Here's how the part is built. I have some questions about the finished solid (model axes, mm). Coordinates: 2 decimals unless noted, no trailing zeros. Loops run counter-clockwise (first coordinate to the right, second up) from the corner with the lowest first, then second, coordinate; pieces in that order, holes last. Notation, with made-up numbers: M -24,49.25 L 1,49.25 A22 cw 1,83.25 Z; hole C -10,61.5 d2. An arc over 180 degrees is marked long. Use one line per item in the form item = value. Start each with the question number.
(1) Please list where these lines run through material, in increasing order: L1, parallel to X at y = 127.5, z = 2.5; L2, parallel to Y at x = 110, z = 8; L3, parallel to X at y = 128.5, z = 6.25.
(2) Imagine slicing it at A-A, the plane x = 55. Please give me the cut outline in (y, z).
(3) Imagine slicing it at B-B, the plane z = 2.75. Please give me the cut outline in (x, y), and give its area (3 significant figures).
(4) Imagine slicing it at C-C, the plane y = 71.5. Please give me the cut outline in (x, z), and give its area (3 significant figures).
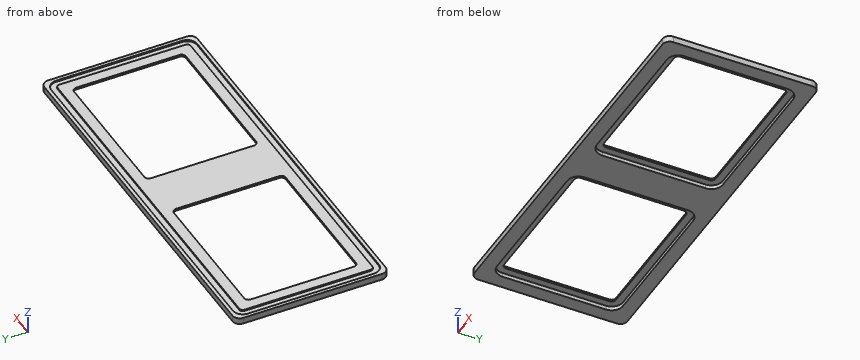
```python
from build123d import *

# Parameters (mm, degrees)
BOSS_EXTRUDE1_DEPTH = 9
CUT_EXTRUDE1_DEPTH  = 2
CUT_EXTRUDE2_DEPTH  = 9
CUT_EXTRUDE4_DEPTH  = 6


with BuildPart() as part:
    # Sketch1 → Boss-Extrude1 (new body)
    with BuildSketch(Plane.XY):
        with BuildLine():
            Line((259.35, -9), (-259.35, -9))
            ThreePointArc((-259.35, -9), (-266.421067812, -6.071067812), (-269.35, 1))
            Line((-269.35, 1), (-269.35, 196.4))
            ThreePointArc((-269.35, 196.4), (-266.421067812, 203.471067812), (-259.35, 206.4))
            Line((-259.35, 206.4), (259.35, 206.4))
            ThreePointArc((259.35, 206.4), (266.421067812, 203.471067812), (269.35, 196.4))
            Line((269.35, 196.4), (269.35, 1))
            ThreePointArc((269.35, 1), (266.421067812, -6.071067812), (259.35, -9))
        make_face()
    extrude(amount=BOSS_EXTRUDE1_DEPTH)

    # Sketch4 → Cut-Extrude1 (cut)
    with BuildSketch(Plane.XY.offset(9)):
        with BuildLine():
            Line((-250.35, -4), (250.35, -4))
            ThreePointArc((250.35, -4), (260.249494937, 0.100505063), (264.35, 10))
            Line((264.35, 10), (264.35, 187.4))
            ThreePointArc((264.35, 187.4), (260.249494937, 197.299494937), (250.35, 201.4))
            Line((250.35, 201.4), (-250.35, 201.4))
            ThreePointArc((-250.35, 201.4), (-260.249494937, 197.299494937), (-264.35, 187.4))
            Line((-264.35, 187.4), (-264.35, 10))
            ThreePointArc((-264.35, 10), (-260.249494937, 0.100505063), (-250.35, -4))
        make_face()
        with BuildLine():
            Line((-250.35, 5), (250.35, 5))
            ThreePointArc((250.35, 5), (253.885533906, 6.464466094), (255.35, 10))
            Line((255.35, 10), (255.35, 187.4))
            ThreePointArc((255.35, 187.4), (253.885533906, 190.935533906), (250.35, 192.4))
            Line((250.35, 192.4), (-250.35, 192.4))
            ThreePointArc((-250.35, 192.4), (-253.885533906, 190.935533906), (-255.35, 187.4))
            Line((-255.35, 187.4), (-255.35, 10))
            ThreePointArc((-255.35, 10), (-253.885533906, 6.464466094), (-250.35, 5))
        make_face(mode=Mode.SUBTRACT)
    extrude(amount=-CUT_EXTRUDE1_DEPTH, mode=Mode.SUBTRACT)

    # Sketch5 → Cut-Extrude2 (cut)
    with BuildSketch(Plane.XY):
        with BuildLine():
            Line((-234.35, 177.4), (-40.731266216, 177.4))
            ThreePointArc((-40.731266216, 177.4), (-36.488625529, 175.642640687), (-34.731266216, 171.4))
            Line((-34.731266216, 171.4), (-34.731266216, 26))
            ThreePointArc((-34.731266216, 26), (-36.488625529, 21.757359313), (-40.731266216, 20))
            Line((-40.731266216, 20), (-234.35, 20))
            ThreePointArc((-234.35, 20), (-238.592640687, 21.757359313), (-240.35, 26))
            Line((-240.35, 26), (-240.35, 171.4))
            ThreePointArc((-240.35, 171.4), (-238.592640687, 175.642640687), (-234.35, 177.4))
        make_face()
    cut_extrude2 = extrude(amount=CUT_EXTRUDE2_DEPTH, mode=Mode.SUBTRACT)

    # Sketch7 → Cut-Extrude4 (cut)
    with BuildSketch(Plane(origin=(0, 0, 0), x_dir=(-1, 0, 0), z_dir=(0, 0, -1))):
        with BuildLine():
            Line((250.35, 26), (250.35, 171.4))
            ThreePointArc((250.35, 171.4), (245.663708499, 182.713708499), (234.35, 187.4))
            Line((234.35, 187.4), (40.731266216, 187.4))
            ThreePointArc((40.731266216, 187.4), (29.417557717, 182.713708499), (24.731266216, 171.4))
            Line((24.731266216, 171.4), (24.731266216, 26))
            ThreePointArc((24.731266216, 26), (29.417557717, 14.686291501), (40.731266216, 10))
            Line((40.731266216, 10), (234.35, 10))
            ThreePointArc((234.35, 10), (245.663708499, 14.686291501), (250.35, 26))
        make_face()
    cut_extrude4 = extrude(amount=-CUT_EXTRUDE4_DEPTH, mode=Mode.SUBTRACT)

    # Mirror1: Cut-Extrude2, Cut-Extrude4 across plane
    add(cut_extrude2.mirror(Plane(origin=(0, 0, 0), x_dir=(0, 0, 1), z_dir=(1, 0, 0))), mode=Mode.SUBTRACT)
    add(cut_extrude4.mirror(Plane(origin=(0, 0, 0), x_dir=(0, 0, 1), z_dir=(1, 0, 0))), mode=Mode.SUBTRACT)


solid = part.part
```
Answer:
q1.L1 = -269.35 to -250.35, -24.73 to 24.73, 250.35 to 269.35
q1.L2 = -9 to -4, 5 to 20, 177.4 to 192.4, 201.4 to 206.4
q1.L3 = -269.35 to -240.35, -34.73 to 34.73, 240.35 to 269.35
q2.outline = M -9,0 L 10,0 L 10,6 L 20,6 L 20,9 L 5,9 L 5,7 L -4,7 L -4,9 L -9,9 Z; M 177.4,6 L 187.4,6 L 187.4,0 L 206.4,0 L 206.4,9 L 201.4,9 L 201.4,7 L 192.4,7 L 192.4,9 L 177.4,9 Z
q3.outline = M -269.35,1 A10 ccw -259.35,-9 L 259.35,-9 A10 ccw 269.35,1 L 269.35,196.4 A10 ccw 259.35,206.4 L -259.35,206.4 A10 ccw -269.35,196.4 Z; hole M -250.35,26 A16 ccw -234.35,10 L -40.73,10 A16 ccw -24.73,26 L -24.73,171.4 A16 ccw -40.73,187.4 L -234.35,187.4 A16 ccw -250.35,171.4 Z; hole M 24.73,26 A16 ccw 40.73,10 L 234.35,10 A16 ccw 250.35,26 L 250.35,171.4 A16 ccw 234.35,187.4 L 40.73,187.4 A16 ccw 24.73,171.4 Z
q3.area = 36,300 mm²
q4.outline = M -269.35,0 L -250.35,0 L -250.35,6 L -240.35,6 L -240.35,9 L -255.35,9 L -255.35,7 L -264.35,7 L -264.35,9 L -269.35,9 Z; M -34.73,6 L -24.73,6 L -24.73,0 L 24.73,0 L 24.73,6 L 34.73,6 L 34.73,9 L -34.73,9 Z; M 240.35,6 L 250.35,6 L 250.35,0 L 269.35,0 L 269.35,9 L 264.35,9 L 264.35,7 L 255.35,7 L 255.35,9 L 240.35,9 Z
q4.area = 871 mm²
